Geometry: final body of the model. Coordinates: model frame, mm. Face numbers are marked on the shaded views. A direction names the side the tool comes from. Round coordinates to 2 decimals unless told otherwise and drop trailing zeros. Order: outer loops, then holes, each group sorted by start corner. A loop starts at its lowest first (then second) coordinate and runs counter-clockwise, first axis right, second up. Notation, with made-up numbers: (14, 43.25) - (37, 43.25) arc R21 cw to (37, 80.25) - close; hole circle Ø5 at (-7.5, 12). An arc over 180 degrees is marked (long way). Put each result on its own line as item: value. Start each with the question number.
(1) Section B-B (x = 6.25). Output: boundary loops of the cut face in (y, z).
(2) Pin query (flat end, axial travel): P1, Ø3, axis at x = 7.5, y = -9.5, coming from the +Z side; P2, Ø1, axis at x = 7.5, y = -4, coming from the +Z side; P3, Ø4, axis at x = 0.5, y = -2, coming from the +Z side. Return the tip coordinate at first contact, or that it passes through.
(3) Access query for the marked faces 1, 2 and 3. Directions: +Z, -Z, +X, -X, +Y, -Y. A direction counts if a zero-diameter tool reaches every point of the face in a straight line with its end or side. Return the directions, or none.
(4) Pull-direction query (X, two-part tool) for the marked faces 4, 5 and 6; classes: released by +X, released by -X, zero draft, split by the parting line, or undercut.
(5) Section C-C (z = 2). Output: boundary loops of the cut face in (x, y).
(6) Section A-A (y = -7.75). Output: boundary loops of the cut face in (x, z), and give its area (3 significant figures).
(7) Section D-D (y = -4.5). Output: boundary loops of the cut face in (x, z), and give its area (3 significant figures).
(8) Material intervals for L1, parallel to Z at x = 3.75, y = -6; L2, parallel to Z at x = -3, y = 0.25; L3, parallel to X at y = -2, z = 4.75, sorted ascending. Write a range as [from, to].
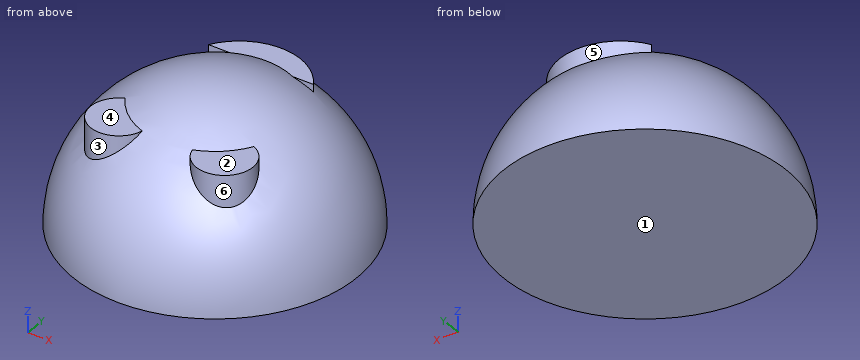
from build123d import *

# Parameters (mm, degrees)
F1_ANGLE = 180
F2_R     = 2.54
F4_DEPTH = 10.8204


with BuildPart() as f1:
    # F0 (on Top) → F1 (revolve)
    with BuildSketch(Plane.XY):
        with BuildLine():
            Line((0, 0), (0, 12.7))
            ThreePointArc((0, 12.7), (-12.7, 0), (0, -12.7))
            Line((0, -12.7), (0, 0))
        make_face()
    revolve(axis=Axis((0, 0, 0), (0, 1, 0)), revolution_arc=F1_ANGLE)

    # F3 (on Top) + F2 (on Top) → F4 (join)
    with BuildSketch(Plane.XY):
        with BuildLine():
            Line((-4.6839732677, 6.046992261), (4.7185341828, 5.9900078923))
            ThreePointArc((4.7185341828, 5.9900078923), (0.0333416464, 8.6686206572), (-4.6839732677, 6.046992261))
        make_face()
    with BuildSketch(Plane.XY):
        with Locations((4.695169162, -5.6601171382)):
            Circle(F2_R)
        with Locations((-4.7209146433, -5.6601171382)):
            Circle(F2_R)
    extrude(amount=F4_DEPTH)


solid = f1.part
Checks:
1. outline: (-11.06, 0) - (11.06, 0) arc R11.06 ccw to (-3.65, 10.44) - (-3.65, 10.82) - (-7.67, 10.82) - (-7.67, 7.96) arc R11.06 ccw to start
2. P1: stops at z = 6.99
2. P2: stops at z = 9.86
2. P3: stops at z = 12.7
3. face 1: -Z, +X, -X, +Y, -Y
3. face 2: +Z, +X, -Y
3. face 3: +Z
4. face 4: zero draft
4. face 5: split by the parting line
4. face 6: undercut
5. outline: circle Ø25.08 at (0, 0)
6. outline: (-10.06, 0) - (10.06, 0) arc R10.06 ccw to (6.14, 7.97) - (6.14, 10.82) - (3.25, 10.82) - (3.25, 9.52) arc R10.06 ccw to (-3.28, 9.51) - (-3.28, 10.82) - (-6.16, 10.82) - (-6.16, 7.95) arc R10.06 ccw to start
6. area: 170 mm²
7. outline: (-11.88, 0) - (11.88, 0) arc R11.88 ccw to (6.95, 9.63) - (6.95, 10.82) - (4.89, 10.82) arc R11.88 ccw to (-4.89, 10.82) - (-6.98, 10.82) - (-6.98, 9.61) arc R11.88 ccw to start
7. area: 224 mm²
8. L1: z = [0, 10.82]
8. L2: z = [0, 12.34]
8. L3: x = [-11.61, 11.61]
